Model file for the job. Use its own axes, mm. Round coordinates to 2 decimals unless told otherwise and drop trailing zeros. Order: outer loops, then holes, each group sorted by start corner. A loop starts at its lowest first (then second) coordinate and runs counter-clockwise, first axis right, second up. Notation, with made-up numbers: (-0.75, 19) - (25.25, 19) arc R22 cw to (25.25, 43) - close; hole circle Ø3 at (-18, 4.5). An arc over 180 degrees is marked (long way). Use one line per item in the form item = value.
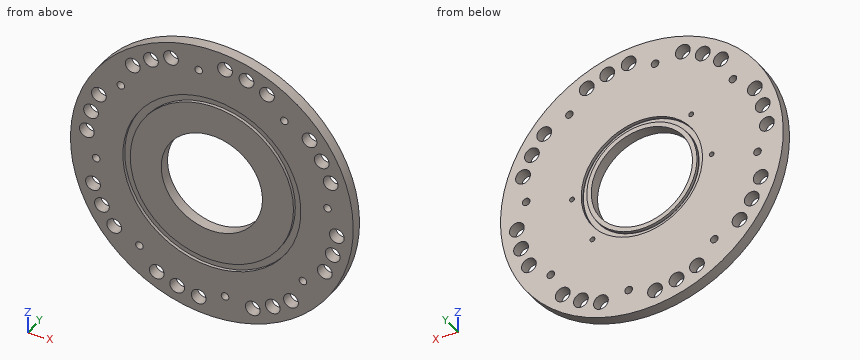
from build123d import *

# Parameters (mm, degrees)
SKETCH1_R                            = 121.5
SKETCH1_R_2                          = 43.5
BOSS_EXTRUDE1_DEPTH                  = 9.525
CUT_EXTRUDE1_START                   = 9.525
SKETCH1_4_R                          = 52.1208
SKETCH1_4_R_2                        = 47.371
CUT_EXTRUDE1_DEPTH                   = 2.8448
CIRPATTERN1_COUNT                    = 16
SKETCH5_R                            = 6.35
CUBE_5_16_CLEARANCE_THRU_HOLES_DEPTH = 173.090748226
F_5_16_18_TAPPED_HOLE1_D             = 6.5278
CIRPATTERN3_COUNT                    = 8
BOTTOM_ISO160_R                      = 76.5
BOTTOM_ISO160_R_2                    = 70.1548
CUT_EXTRUDE3_DEPTH                   = 2.79
FILLET1_R                            = 0.254


with BuildPart() as part:
    # Sketch1 → Boss-Extrude1 (new body)
    with BuildSketch(Plane(origin=(0, 0, 0), x_dir=(1, 0, 0), z_dir=(0, 1, 0))):
        with Locations(Location((0, 0, 0), (0, 0, 90))):
            Circle(SKETCH1_R)
        with Locations(Location((0, 0, 0), (0, 0, 90))):
            Circle(SKETCH1_R_2, mode=Mode.SUBTRACT)
    extrude(amount=BOSS_EXTRUDE1_DEPTH)

    # Sketch1<4> → Cut-Extrude1 (cut)
    with BuildSketch(Plane(origin=(0, 0, 0), x_dir=(1, 0, 0), z_dir=(0, 1, 0)).offset(CUT_EXTRUDE1_START)):
        with Locations(Location((0, 0, 0), (0, 0, 270))):
            Circle(SKETCH1_4_R)
        with Locations(Location((0, 0, 0), (0, 0, 270))):
            Circle(SKETCH1_4_R_2, mode=Mode.SUBTRACT)
    extrude(amount=-CUT_EXTRUDE1_DEPTH, mode=Mode.SUBTRACT)

    # Sketch4 → M5x0.8 Tapped Hole2 (revolve, cut)
    with BuildSketch(Plane(origin=(60, 9.525, 0), x_dir=(0, 0, 1), z_dir=(1, 0, 0))):
        Polygon((0, 0), (0, 7), (2.1, 5.7381927), (2.1, 0), align=None)
    m5x0_8_tapped_hole2 = revolve(axis=Axis((60, 15.875, 0), (0, -1, 0)), mode=Mode.SUBTRACT)

    # CirPattern1: M5x0.8 Tapped Hole2 ×16 about axis, 12 skipped
    cirpattern1_axis = Axis((0, 9.525, 0), (0, -1, 0))
    add([m5x0_8_tapped_hole2.rotate(cirpattern1_axis, i * 360 / CIRPATTERN1_COUNT) for i in range(1, CIRPATTERN1_COUNT) if i not in (1, 2, 3, 4, 5, 7, 9, 10, 11, 12, 13, 15)], mode=Mode.SUBTRACT)

    # Sketch5 → Cube_5/16_Clearance_Thru Holes (cut, through all)
    with BuildSketch(Plane(origin=(0, 0, 0), x_dir=(1, 0, 0), z_dir=(0, 1, 0))):
        with Locations(Location((103.816263161, 29.768834428, 0), (0, 0, 270))):
            Circle(SKETCH5_R)
        with Locations(Location((94.458928371, -52.359438987, 0), (0, 0, 270))):
            Circle(SKETCH5_R)
        with Locations(Location((29.768834428, -103.816263161, 0), (0, 0, 270))):
            Circle(SKETCH5_R)
        with Locations(Location((-52.359438987, -94.458928371, 0), (0, 0, 270))):
            Circle(SKETCH5_R)
        with Locations(Location((-103.816263161, -29.768834428, 0), (0, 0, 270))):
            Circle(SKETCH5_R)
        with Locations(Location((-94.458928371, 52.359438987, 0), (0, 0, 270))):
            Circle(SKETCH5_R)
        with Locations(Location((52.359438987, 94.458928371, 0), (0, 0, 270))):
            Circle(SKETCH5_R)
        with Locations(Location((-29.768834428, 103.816263161, 0), (0, 0, 270))):
            Circle(SKETCH5_R)
        with Locations(Location((11.289074033, -107.4083647, 0), (0, 0, 270))):
            Circle(SKETCH5_R)
        with Locations(Location((47.344083853, -97.069757, 0), (0, 0, 270))):
            Circle(SKETCH5_R)
        with Locations(Location((83.931763837, -67.966602233, 0), (0, 0, 270))):
            Circle(SKETCH5_R)
        with Locations(Location((102.116006165, -35.161360681, 0), (0, 0, 270))):
            Circle(SKETCH5_R)
        with Locations(Location((107.4083647, 11.289074033, 0), (0, 0, 270))):
            Circle(SKETCH5_R)
        with Locations(Location((97.069757, 47.344083853, 0), (0, 0, 270))):
            Circle(SKETCH5_R)
        with Locations(Location((-35.161360681, -102.116006165, 0), (0, 0, 270))):
            Circle(SKETCH5_R)
        with Locations(Location((-67.966602233, -83.931763837, 0), (0, 0, 270))):
            Circle(SKETCH5_R)
        with Locations(Location((-107.4083647, -11.289074033, 0), (0, 0, 270))):
            Circle(SKETCH5_R)
        with Locations(Location((-97.069757, -47.344083853, 0), (0, 0, 270))):
            Circle(SKETCH5_R)
        with Locations(Location((-102.116006165, 35.161360681, 0), (0, 0, 270))):
            Circle(SKETCH5_R)
        with Locations(Location((-83.931763837, 67.966602233, 0), (0, 0, 270))):
            Circle(SKETCH5_R)
        with Locations(Location((35.161360681, 102.116006165, 0), (0, 0, 270))):
            Circle(SKETCH5_R)
        with Locations(Location((67.966602233, 83.931763837, 0), (0, 0, 270))):
            Circle(SKETCH5_R)
        with Locations(Location((-11.289074033, 107.4083647, 0), (0, 0, 270))):
            Circle(SKETCH5_R)
        with Locations(Location((-47.344083853, 97.069757, 0), (0, 0, 270))):
            Circle(SKETCH5_R)
    extrude(amount=CUBE_5_16_CLEARANCE_THRU_HOLES_DEPTH, mode=Mode.SUBTRACT)

    # 5/16-18 Tapped Hole1 (through all)
    with Locations(Plane(origin=(-62.251463664, 0, -78.260815685), x_dir=(0, 0, -1), z_dir=(0, -1, 0))):
        with Locations((0, 0)):
            f_5_16_18_tapped_hole1 = Hole(F_5_16_18_TAPPED_HOLE1_D / 2)

    # CirPattern3: 5/16-18 Tapped Hole1 ×8 about axis
    cirpattern3_axis = Axis((0, 0, 0), (0, 1, 0))
    for i in range(1, CIRPATTERN3_COUNT):
        add(f_5_16_18_tapped_hole1.rotate(cirpattern3_axis, i * 360 / CIRPATTERN3_COUNT), mode=Mode.SUBTRACT)

    # Bottom_Iso160 → Cut-Extrude3 (cut)
    with BuildSketch(Plane(origin=(0, 0, 0), x_dir=(1, 0, 0), z_dir=(0, 1, 0))):
        with Locations(Location((0, 0, 0), (0, 0, 270))):
            Circle(BOTTOM_ISO160_R)
        with Locations(Location((0, 0, 0), (0, 0, 270))):
            Circle(BOTTOM_ISO160_R_2, mode=Mode.SUBTRACT)
    extrude(amount=CUT_EXTRUDE3_DEPTH, mode=Mode.SUBTRACT)

    # Fillet1
    fillet1_edges = [part.edges().sort_by_distance(p)[0] for p in [
        (0, 6.6802, -52.1208),
        (0, 6.6802, -47.371),
    ]]
    fillet(fillet1_edges, radius=FILLET1_R)


solid = part.part
(1) Slice it at A-A on x = 0. Give the cut face in (y, z) (3 decimals), then the cut area to 3 significant figures.
Report:
outline = (0, -121.5) - (9.525, -121.5) - (9.525, -52.121) - (6.934, -52.121) arc R0.254 cw to (6.68, -51.867) - (6.68, -47.625) arc R0.254 cw to (6.934, -47.371) - (9.525, -47.371) - (9.525, -43.5) - (0, -43.5) - (0, -70.155) - (2.79, -70.155) - (2.79, -76.5) - (0, -76.5) - close; (0, 43.5) - (9.525, 43.5) - (9.525, 47.371) - (6.934, 47.371) arc R0.254 cw to (6.68, 47.625) - (6.68, 51.867) arc R0.254 cw to (6.934, 52.121) - (9.525, 52.121) - (9.525, 121.5) - (0, 121.5) - (0, 76.5) - (2.79, 76.5) - (2.79, 70.155) - (0, 70.155) - close
area = 1,420 mm2
(2) Pin check, flat tips, straight feed: pin 1 (2.5 mm diameter, centred on x = -60, z = 0, fed in from +Y); pin 2 (6 mm diameter, centred on x = 11.32, z = -99.36, fed in from -Y); pin 3 (2 mm diameter, centred on x = -44.5, y = 8, fed in from -Z); pin 4 (4 mm diameter, centred on y = 5, z = 21, fed in from +X). Stop position of each tip, or through.
Report:
pin_1 = 3.28
pin_2 = through
pin_3 = -113.45
pin_4 = 120.01
(3) Probe probe 1 along Z at (x, y) = (31.5, 1); probe 2 along X at (y, z) = (3, -39); probe 3 along Z at (x, y) = (26.5, 1.25). List the from-to ranges inside material, lowest first. Write a range as [from, to].
Report:
probe_1 = [-117.35, -107.3], [-96.93, -69.71], [-62.69, -30], [30, 62.69], [69.71, 97.71], [109.93, 117.35]
probe_2 = [-115.07, -107.17], [-97.06, -19.27], [19.27, 115.07]
probe_3 = [-118.57, -71.76], [-64.96, -34.5], [34.5, 64.96], [71.76, 98.37], [109.26, 118.57]
(4) Slice it at B-B on y = 5.25. Count the separate pieces of the cut face and the enclosed holes in it, then the cut area to 3 significant figures.
Report:
separate_pieces = 1
enclosed_holes = 37
area = 37,100 mm2
